```python
from build123d import *

# Parameters (mm, degrees)
RECPAT_COUNT = 2
RECPAT_ANGLE = 90


with BuildPart() as part:
    # Fillet1: read off the stored shape, not the designer's step
    # Fillet1 outline → Fillet1 (revolve)
    with BuildSketch(Plane.YX):
        with BuildLine():
            Line((1.5, 2.45), (1.5, 22.35))
            Line((1.5, 22.35), (0, 22.35))
            Line((0, 22.35), (0, 1.65))
            Line((0, 1.65), (3.75, 1.65))
            Line((3.75, 1.65), (3.75, 2.35))
            Line((3.75, 2.35), (1.6, 2.35))
            ThreePointArc((1.6, 2.35), (1.529289322, 2.379289322), (1.5, 2.45))
        make_face()
    revolve(axis=Axis((0, 0, 0), (1, 0, 0)))

    # PanSke → Pan (revolve)
    with BuildSketch(Plane.XY, mode=Mode.PRIVATE) as pan_sk:
        with BuildLine():
            Line((1.65, 3.133289007), (1.65, 0))
            Line((1.65, 0), (0, 0))
            ThreePointArc((0, 0), (0.437709114, 1.770593121), (1.65, 3.133289007))
        make_face()
    revolve(pan_sk.sketch.rotate(Axis((0, 0, 0), (1, 0, 0)), 90), axis=Axis((0, 0, 0), (1, 0, 0)))

    # Sketch3 → Recess section 0
    with BuildSketch(Plane(origin=(0, 0, 0), x_dir=(0, 0, -1), z_dir=(1, 0, 0))):
        with BuildLine():
            Line((-0.37, 1.45), (0.37, 1.45))
            Line((0.37, 1.45), (0.37, -1.45))
            Line((0.37, -1.45), (-0.37, -1.45))
            Line((-0.37, -1.45), (-0.37, 1.45))
        make_face()
    # Sketch4 → Recess section 1
    with BuildSketch(Plane(origin=(1.83, 0, 0), x_dir=(0, 0, -1), z_dir=(1, 0, 0))):
        with BuildLine():
            Line((-0.37, 2.106524682), (0.37, 2.106524682))
            Line((0.37, 2.106524682), (0.37, -2.106524682))
            Line((0.37, -2.106524682), (-0.37, -2.106524682))
            Line((-0.37, -2.106524682), (-0.37, 2.106524682))
        make_face()
    recess = loft(mode=Mode.SUBTRACT)

    # RecPat: Recess ×2 about axis
    recpat_axis = Axis((0, 0, 0), (1, 0, 0))
    for i in range(1, RECPAT_COUNT):
        add(recess.rotate(recpat_axis, i * RECPAT_ANGLE / (RECPAT_COUNT - 1)), mode=Mode.SUBTRACT)

    # RecCorSke → RecessCore (revolve, cut)
    with BuildSketch(Plane.XY, mode=Mode.PRIVATE) as recesscore_sk:
        Polygon((0, 0), (0, 0.877663335), (4.6, 0.556), (4.780655351, 0), align=None)
    revolve(recesscore_sk.sketch.rotate(Axis((-3.175, 0, 0), (1, 0, 0)), 90), axis=Axis((-3.175, 0, 0), (1, 0, 0)), mode=Mode.SUBTRACT)


solid = part.part
```
Read the model definition and answer for the solid it produces. Units are mm, in the model's axes. Coordinates: 2 decimals unless noted, no trailing zeros. Write each loop counter-clockwise with the first axis right and the second up, starting at its lowest first coordinate (ties: lowest second). Pieces come first, ordered by that corner, then holes. Notation, with made-up numbers: (-39.75, 5) - (-20.75, 5) arc R17 ccw to (-20.75, 26) - close; hole circle Ø9 at (87.5, 70). An arc over 180 degrees is marked (long way). Answer as a JSON object with one key per item and string values. Group by question number.
1. Consider L1, parallel to X at y = -2.5, z = 2.5; L2, parallel to X at y = -0.25, z = -1.25; L3, parallel to Y at x = 8, z = 1.25. Determine where each line is inside the solid, lowest interval first. Write a range as [from, to].
2. A cutting plane is placed at A-A (x = 9). Determine the outline of the cut face in (y, z), plus the area to 3 significant figures.
3. A cutting plane is placed at B-B (y = -2.5). Determine the outline of the cut face in (x, z), plus the area to 3 significant figures.
4. The mould has two halves that part along Y. Classify faces 1 (the conical face through (4.77, -0.03, 0)), 2 (the flat face through (2.35, 0, -2)), 3 (the cylindrical face through (12.54, -1.5, 0.07)), 4 (the conical face through (2.882, -0.457, -0.498)): +Y half, -Y half, draft (parallel to the pull), parting line (faces both ways), or undercut.
5. Each of these flat-tipped pins is pushed along its axis until it touches: P1, Ø0.6, axis at y = 0, z = -1, coming from the -X side; P2, Ø4, axis at x = 8.5, z = 1, coming from the -Y side; P3, Ø2, axis at y = 1.5, z = -2, coming from the -X side; P4, Ø2, axis at x = 5.5, y = -3, coming from the +Z side. Where does it stop, or does it pass through?
Worked out:
{
 "1": {"L1": "x = [1.65, 2.35]", "L2": "x = [1.83, 22.35]", "L3": "y = [-0.83, 0.83]"},
 "2": {"outline": "circle Ø3 at (0, 0)", "area": "7.07 mm²"},
 "3": {"outline": "(1.65, -2.8) - (2.35, -2.8) - (2.35, 2.8) - (1.65, 2.8) - (1.65, 1.89) arc R2.86 ccw to (1.65, -1.89) - close", "area": "5.76 mm²"},
 "4": {"face 1": "undercut", "face 2": "draft", "face 3": "parting line", "face 4": "undercut"},
 "5": {"P1": "stops at x = 1.83", "P2": "stops at y = -1.5", "P3": "stops at x = 0.31", "P4": "passes through"}
}
